Here's how the part is built. I have some questions about the finished solid (model axes, mm). A direction names the side the tool comes from. Round coordinates to 2 decimals unless told otherwise and drop trailing zeros. Write each loop counter-clockwise with the first axis right and the second up, starting at its lowest first coordinate (ties: lowest second). Pieces come first, ordered by that corner, then holes. Notation, with made-up numbers: (21, -12) -> (38, -12) arc R17 ccw to (38, -5) -> close; hole circle Ø6 at (-4, 25). An arc over 180 degrees is marked (long way). Put each result on its own line as item: value. Start each with the question number.
1) Which directions (+Z, -Z, +X, -X, +Y, -Y) give clear straight access to the entire face, cutting with the end or side of a thin tool? Please do faces 1 (the flat face through (35, -4, 20)), 2 (the cylindrical face through (7.973, -1.455, 24.65)).
2) I want a section at D-D, the plane z = 26. List the corners of the cut face in (x, y) for me, then the cut area to 3 significant figures.
3) I want a section at A-A, the plane z = 5. List the corners of the cut face in (x, y) for me, then the cut area to 3 significant figures.
4) If I drill on line 1 along X through (y, z) = (-0.5, 2); line 2 along Y through (x, z) = (22, 18); line 3 along Y through (x, z) = (40.5, 7), over which ranges is the centre line in solid material (lowest first)? Write a range as [from, to].
5) I want a section at C-C, the plane x = 47. List the corners of the cut face in (y, z) for me, then the cut area to 3 significant figures.
6) We'd pull the mould along Y, two halves only. Please class faces 3 (the flat face through (7.9, -13, 25)), 4 (the cylindrical face through (34.995, -10.444, 42.395)), 5 (the flat face through (35, 5, 42)): released by +Y, released by -Y, zero draft, split by the parting line, or undercut.
7) I want a section at B-B, the plane y = 0. List the corners of the cut face in (x, z) for me, then the cut area to 3 significant figures.
8) Will these pins go through, and if not, where does the flat tip stop? P1, Ø2.5, axis at x = 46.09, z = 45, coming from the -Y side; P2, Ø3, axis at x = 47.5, z = 6, coming from the +Y side; P3, Ø3, axis at y = 2, z = 29.5, coming from the -X side; P4, Ø10, axis at x = 17, z = 41.5, coming from the +Y side.
from build123d import *

# Parameters (mm, degrees)
BOSS_EXTRUDE1_DEPTH = 50
SKETCH2_W           = 15
SKETCH2_H           = 20.436302067
CUT_EXTRUDE1_DEPTH  = 20
SKETCH3_R           = 2
CUT_EXTRUDE2_DEPTH  = 76.033433569


with BuildPart() as part:
    # Sketch1 → Boss-Extrude1 (new body)
    with BuildSketch(Plane.XY):
        with BuildLine():
            Line((34.065465836, 5), (36.21714256, 5))
            ThreePointArc((36.21714256, 5), (37.036070696, -1.364788891), (35.046720745, -7.465909091))
            ThreePointArc((35.046720745, -7.465909091), (35.016915208, -10.48285658), (37.624814048, -12))
            Line((37.624814048, -12), (53.301183412, -12))
            Line((53.301183412, -12), (53.301183412, -15))
            Line((53.301183412, -15), (7.9, -15))
            Line((7.9, -15), (7.9, -11.953738346))
            ThreePointArc((7.9, -11.953738346), (10.103218459, -10.248134062), (9.953279255, -7.465909091))
            ThreePointArc((9.953279255, -7.465909091), (7.963929304, -1.364788891), (8.78285744, 5))
            Line((8.78285744, 5), (10.934534164, 5))
            ThreePointArc((10.934534164, 5), (22.5, -12.6), (34.065465836, 5))
        make_face()
    extrude(amount=BOSS_EXTRUDE1_DEPTH)

    # Sketch2 → Cut-Extrude1 (cut)
    with BuildSketch(Plane(origin=(53.301183412, 0, 0), x_dir=(0, 0, -1), z_dir=(1, 0, 0))):
        with Locations((-27.5, -1.781848967)):
            Rectangle(SKETCH2_W, SKETCH2_H)
    extrude(amount=-CUT_EXTRUDE1_DEPTH, mode=Mode.SUBTRACT)

    # Sketch3 → Cut-Extrude2 (cut, through all)
    with BuildSketch(Plane(origin=(0, -12, 0), x_dir=(1, 0, 0), z_dir=(0, 1, 0))):
        with Locations(Location((46.094817468, -45, 0), (0, 0, 180))):
            Circle(SKETCH3_R)
        with Locations(Location((46.094817468, -5, 0), (0, 0, 180))):
            Circle(SKETCH3_R)
    extrude(amount=-CUT_EXTRUDE2_DEPTH, mode=Mode.SUBTRACT)


solid = part.part
Findings:
1. face 1: +X, +Y
1. face 2: +Z, -Z, -X
2. outline: (7.9, -15) -> (53.3, -15) -> (53.3, -12) -> (33.3, -12) -> (33.3, -6.49) arc R12.6 cw to (10.93, 5) -> (8.78, 5) arc R14.6 ccw to (9.95, -7.47) arc R3 cw to (7.9, -11.95) -> close
2. area: 196 mm2
3. outline: (7.9, -15) -> (44.09, -15) -> (44.09, -12) -> (37.62, -12) arc R3 cw to (35.05, -7.47) arc R14.6 ccw to (36.22, 5) -> (34.07, 5) arc R12.6 cw (long way) to (10.93, 5) -> (8.78, 5) arc R14.6 ccw to (9.95, -7.47) arc R3 cw to (7.9, -11.95) -> close; (48.09, -15) -> (53.3, -15) -> (53.3, -12) -> (48.09, -12) -> close
3. area: 218 mm2
4. line 1: x = [7.91, 9.91], [35.09, 37.09]
4. line 2: y = [-15, -12.59]
4. line 3: y = [-15, -12]
5. outline: (-15, 0) -> (-12, 0) -> (-12, 3.22) -> (-15, 3.22) -> close; (-15, 6.78) -> (-12, 6.78) -> (-12, 43.22) -> (-15, 43.22) -> close; (-15, 46.78) -> (-12, 46.78) -> (-12, 50) -> (-15, 50) -> close
5. area: 129 mm2
6. face 3: zero draft
6. face 4: undercut
6. face 5: released by +Y
7. outline: (7.9, 0) -> (9.9, 0) -> (9.9, 50) -> (7.9, 50) -> close; (35.1, 0) -> (37.1, 0) -> (37.1, 20) -> (35.1, 20) -> close; (35.1, 35) -> (37.1, 35) -> (37.1, 50) -> (35.1, 50) -> close
7. area: 170 mm2
8. P1: passes through
8. P2: stops at y = -12
8. P3: stops at x = 7.91
8. P4: stops at y = -6.96
